The model under review builds one solid part; all positions refer to its coordinate system, in mm. Face numbers are marked on the shaded views. A direction names the side the tool comes from. Give positions to 0.01 mm unless a question says otherwise; leave off trailing zeros. Loops run counter-clockwise (first coordinate to the right, second up) from the corner with the lowest first, then second, coordinate; pieces in that order, holes last. Notation, with made-up numbers: (-4, -10.5) -> (39, -10.5) arc R21 cw to (39, 20.5) -> close; hole circle Ø8 at (-13.75, 41.5). An arc over 180 degrees is marked (long way). Write each question's results on one line, items separated by ' | '. Start each with the question number.
Q1. Mouldability with a two-part tool opening along Y and no side actions: class the marked faces 4, 5 and 6 as released by +Y, released by -Y, zero draft, split by the parting line, or undercut.
Q2. We need section D-D (y = 35.5). Write out the cut boundary in (x, z), plus the area to 3 significant figures.
Q3. We need section C-C (x = 74). Write out the cut boundary in (y, z), plus the area to 3 significant figures.
Q4. We need section B-B (z = 15). Write out the cut boundary in (x, y).
Q5. Wall thickness on L1, parallel to Z at x = 75.5, y = 13.5; L2, parallel to Y at x = 85, z = 56.5; L3, parallel to Z at x = 40.5, y = 30.5: over which ranges is each line inside the solid? List them lowest first. Write a range as [from, to].
Q6. We need section A-A (y = -0.5). Write out the cut boundary in (x, z).
Q7. Insertion check: pin 1 Ø7 at (x, z) = (33.5, 64) entering from -Y; pin 2 Ø8 at (x, y) = (74.5, -30.5) entering from +Z; pin 3 Ø8 at (x, z) = (17, 60.5) entering from +Y; pin 4 Ø8 at (y, z) = (-29.5, 63) entering from -X. Each pin has a flat end and moves straight along its axis. Give the tip position at first contact, or say it passes through.
Q8. Machinability: for the marked faces 1, 2 and 3, which of the approach directions +Z, -Z, +X, -X, +Y, -Y give a long, thin tool a straight path to every point of the face, cutting with its end or side? Answer none if there is none.
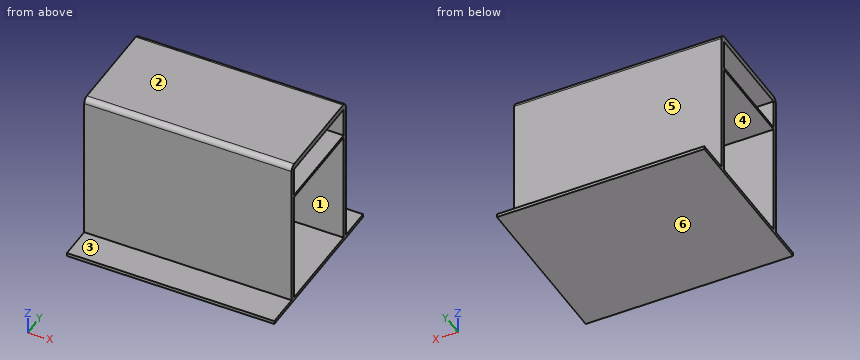
from build123d import *

# Parameters (mm, degrees)
F1_DEPTH = 100
F3_R     = 2.5


with BuildPart() as f1:
    # F0 (on Right) → F1 (new body)
    with BuildSketch(Plane.YZ):
        Polygon((-41, 0), (0, 0), (0, 1.6), (-23, 1.6), (-23, 56.6), (0, 56.6), (0, 57.8), (-23, 57.8), (-23, 72), (0, 72), (0, 74.8), (-25, 74.8), (-25, 1.6), (-41, 1.6), align=None)
    extrude(amount=F1_DEPTH)

    # F2: F1 across plane


with BuildPart() as f1_1:
    add(f1.part)
    add(f1.part.mirror(Plane.XZ))

    # F3
    f3_edges = [f1_1.edges().sort_by_distance(p)[0] for p in [
        (50, -25, 74.8),
        (50, 25, 74.8),
    ]]
    fillet(f3_edges, radius=F3_R)


solid = f1_1.part
Output:
1) face 4: undercut | face 5: released by +Y | face 6: zero draft
2) outline: (0, 0) -> (100, 0) -> (100, 1.6) -> (0, 1.6) -> close | area: 160 mm2
3) outline: (-41, 0) -> (41, 0) -> (41, 1.6) -> (25, 1.6) -> (25, 72.3) arc R2.5 ccw to (22.5, 74.8) -> (-22.5, 74.8) arc R2.5 ccw to (-25, 72.3) -> (-25, 1.6) -> (-41, 1.6) -> close; hole (-23, 1.6) -> (23, 1.6) -> (23, 56.6) -> (-23, 56.6) -> close; hole (-23, 57.8) -> (23, 57.8) -> (23, 72) -> (-23, 72) -> close | area: 605 mm2
4) outline: (0, -25) -> (100, -25) -> (100, -23) -> (0, -23) -> close; (0, 23) -> (100, 23) -> (100, 25) -> (0, 25) -> close
5) L1: [0, 1.6], [56.6, 57.8], [72, 74.8] | L2: [-25, -23], [23, 25] | L3: [0, 1.6]
6) outline: (0, 0) -> (100, 0) -> (100, 1.6) -> (0, 1.6) -> close; (0, 56.6) -> (100, 56.6) -> (100, 57.8) -> (0, 57.8) -> close; (0, 72) -> (100, 72) -> (100, 74.8) -> (0, 74.8) -> close
7) pin 1: y = -25 | pin 2: z = 1.6 | pin 3: y = 25 | pin 4: through
8) face 1: +X, -X | face 2: +Z, +X, -X, +Y, -Y | face 3: +Z, +X, -X, -Y
